```python
from build123d import *

# Parameters (mm, degrees)
EXTRUDE_1_DEPTH          = 10
EXTRUDE_2_DEPTH          = 10
EXTRUDE_3_DEPTH          = 900
SKETCH_4_W               = 40
SKETCH_4_H               = 15
EXTRUDE_4_DEPTH          = 45
CUT_EXTRUDE_1_DEPTH      = 975.114982946
CUT_EXTRUDE_1_DEPTH_BACK = 975.114982946
SKETCH_6_W               = 150
SKETCH_6_H               = 260
EXTRUDE_5_DEPTH          = 20
EXTRUDE_6_DEPTH          = 60
EXTRUDE_7_REACH          = 955.362
SKETCH_8_R               = 15
SKETCH_11_R              = 24
SKETCH_11_R_2            = 18
EXTRUDE_10_DEPTH         = 15
SKETCH_12_W              = 30
SKETCH_12_H              = 860
CUT_EXTRUDE_3_DEPTH      = 10
SKETCH_13_W              = 5
SKETCH_13_H              = 860
EXTRUDE_11_DEPTH         = 5
SKETCH_14_W              = 8
SKETCH_14_H              = 860
EXTRUDE_12_DEPTH         = 3
SKETCH_17_R              = 5
CUT_EXTRUDE_4_DEPTH      = 5
SKETCH_20_W              = 20
SKETCH_20_H              = 20
EXTRUDE_13_DEPTH         = 10
SKETCH_23_W              = 10
SKETCH_23_H              = 10
CUT_EXTRUDE_8_DEPTH      = 20


with BuildPart() as part:
    # 草图1 → 凸台-拉伸1 (new body)
    with BuildSketch(Plane(origin=(0, 0, 0), x_dir=(1, 0, 0), z_dir=(0, 1, 0))):
        Polygon((-150, 50), (-150, 150), (200, 150), (200, -150), (-150, -150), align=None)
    extrude(amount=EXTRUDE_1_DEPTH)

    # 草图2 → 凸台-拉伸2 (add)
    with BuildSketch(Plane(origin=(0, 10, 0), x_dir=(1, 0, 0), z_dir=(0, 1, 0))):
        with BuildLine():
            Line((-100, -20), (-100, 120))
            ThreePointArc((-100, 120), (-94.142135624, 134.142135624), (-80, 140))
            Line((-80, 140), (80, 140))
            ThreePointArc((80, 140), (94.142135624, 134.142135624), (100, 120))
            Line((100, 120), (100, -120))
            ThreePointArc((100, -120), (94.142135624, -134.142135624), (80, -140))
            Line((80, -140), (-80, -140))
            ThreePointArc((-80, -140), (-94.142135624, -134.142135624), (-100, -120))
            Line((-100, -120), (-100, -20))
        make_face()
    extrude(amount=EXTRUDE_2_DEPTH)

    # 草图3 → 凸台-拉伸3 (add)
    with BuildSketch(Plane(origin=(0, 20, 0), x_dir=(1, 0, 0), z_dir=(0, 1, 0))):
        Polygon((-50, 100), (-50, -100), (-50, -130), (-40, -130), (-40, 130), (-50, 130), align=None)
    extrude(amount=EXTRUDE_3_DEPTH)

    # 草图4 → 凸台-拉伸4 (add)
    with BuildSketch(Plane(origin=(0, 20, 0), x_dir=(1, 0, 0), z_dir=(0, 1, 0))):
        with Locations((-70, -92.5)):
            Rectangle(SKETCH_4_W, SKETCH_4_H)
        with Locations((-70, 92.5)):
            Rectangle(SKETCH_4_W, SKETCH_4_H)
    extrude(amount=EXTRUDE_4_DEPTH)

    # 草图5 → 切除-拉伸1 (cut, two sides: drawn at the far end of the back side and taken through both)
    with BuildSketch(Plane(origin=(0, 0, -100), x_dir=(-1, 0, 0), z_dir=(0, 0, -1)).offset(-CUT_EXTRUDE_1_DEPTH_BACK)):
        Polygon((90, 65), (90, 50), (50, 65), align=None)
    extrude(amount=CUT_EXTRUDE_1_DEPTH + CUT_EXTRUDE_1_DEPTH_BACK, mode=Mode.SUBTRACT)

    # 草图6 → 凸台-拉伸5 (add)
    with BuildSketch(Plane(origin=(0, 920, 0), x_dir=(1, 0, 0), z_dir=(0, 1, 0))):
        with Locations((25, 0)):
            Rectangle(SKETCH_6_W, SKETCH_6_H)
    extrude(amount=EXTRUDE_5_DEPTH)

    # 草图7 → 凸台-拉伸6 (add)
    with BuildSketch(Plane(origin=(-40, 0, 0), x_dir=(0, 0, -1), z_dir=(1, 0, 0))):
        Polygon((-95, 920), (-65, 920), (-65, 60), (-65, 20), (-95, 20), (-95, 60), align=None)
        Polygon((95, 920), (65, 920), (65, 60), (65, 20), (95, 20), (95, 60), align=None)
    extrude(amount=EXTRUDE_6_DEPTH)

    # 草图8 → 凸台-拉伸7 (add, up to next)
    with BuildSketch(Plane(origin=(0, 20, 0), x_dir=(1, 0, 0), z_dir=(0, 1, 0)), mode=Mode.PRIVATE) as extrude_7_sk1:
        with Locations(Location((0, 0, 0), (0, 0, 90))):
            Circle(SKETCH_8_R)
    extrude_7_tool1 = extrude(extrude_7_sk1.sketch, amount=EXTRUDE_7_REACH, mode=Mode.PRIVATE) - part.part
    add(extrude_7_tool1.solids().sort_by_distance((0, 20, 0))[0])

    # 草图11 → 凸台-拉伸10 (add)
    with BuildSketch(Plane.XZ.offset(-920)):
        with Locations(Location((0, 0, 0), (0, 0, 90))):
            Circle(SKETCH_11_R)
        with Locations(Location((0, 0, 0), (0, 0, 270))):
            Circle(SKETCH_11_R_2, mode=Mode.SUBTRACT)
    extrude(amount=EXTRUDE_10_DEPTH)

    # 草图12 → 切除-拉伸3 (cut)
    with BuildSketch(Plane(origin=(20, 0, 0), x_dir=(0, 0, -1), z_dir=(1, 0, 0))):
        with Locations((80, 490)):
            Rectangle(SKETCH_12_W, SKETCH_12_H)
        with Locations((-80, 490)):
            Rectangle(SKETCH_12_W, SKETCH_12_H)
    extrude(amount=-CUT_EXTRUDE_3_DEPTH, mode=Mode.SUBTRACT)

    # 草图13 → 凸台-拉伸11 (add)
    with BuildSketch(Plane(origin=(10, 0, 0), x_dir=(0, 0, -1), z_dir=(1, 0, 0))):
        with Locations((-92.5, 490)):
            Rectangle(SKETCH_13_W, SKETCH_13_H)
        with Locations((-67.5, 490)):
            Rectangle(SKETCH_13_W, SKETCH_13_H)
        with Locations((67.5, 490)):
            Rectangle(SKETCH_13_W, SKETCH_13_H)
        with Locations((92.5, 490)):
            Rectangle(SKETCH_13_W, SKETCH_13_H)
    extrude(amount=EXTRUDE_11_DEPTH)

    # 草图14 → 凸台-拉伸12 (add)
    with BuildSketch(Plane(origin=(15, 0, 0), x_dir=(0, 0, -1), z_dir=(1, 0, 0))):
        with Locations((-91, 490)):
            Rectangle(SKETCH_14_W, SKETCH_14_H)
        with Locations((-69, 490)):
            Rectangle(SKETCH_14_W, SKETCH_14_H)
        with Locations((69, 490)):
            Rectangle(SKETCH_14_W, SKETCH_14_H)
        with Locations((91, 490)):
            Rectangle(SKETCH_14_W, SKETCH_14_H)
    extrude(amount=EXTRUDE_12_DEPTH)

    # 草图17 → 切除-拉伸4 (cut)
    with BuildSketch(Plane(origin=(10, 0, 0), x_dir=(0, 0, -1), z_dir=(1, 0, 0))):
        with Locations((-80, 675)):
            Circle(SKETCH_17_R)
        with Locations((-80, 625)):
            Circle(SKETCH_17_R)
        with Locations((-80, 575)):
            Circle(SKETCH_17_R)
        with Locations((-80, 525)):
            Circle(SKETCH_17_R)
        with Locations((-80, 475)):
            Circle(SKETCH_17_R)
        with Locations((-80, 425)):
            Circle(SKETCH_17_R)
        with Locations((-80, 375)):
            Circle(SKETCH_17_R)
        with Locations((-80, 325)):
            Circle(SKETCH_17_R)
        with Locations((-80, 275)):
            Circle(SKETCH_17_R)
        with Locations((-80, 225)):
            Circle(SKETCH_17_R)
        with Locations((-80, 175)):
            Circle(SKETCH_17_R)
        with Locations((-80, 125)):
            Circle(SKETCH_17_R)
        with Locations((-80, 75)):
            Circle(SKETCH_17_R)
        with Locations((80, 675)):
            Circle(SKETCH_17_R)
        with Locations((80, 625)):
            Circle(SKETCH_17_R)
        with Locations((80, 575)):
            Circle(SKETCH_17_R)
        with Locations((80, 525)):
            Circle(SKETCH_17_R)
        with Locations((80, 475)):
            Circle(SKETCH_17_R)
        with Locations((80, 425)):
            Circle(SKETCH_17_R)
        with Locations((80, 375)):
            Circle(SKETCH_17_R)
        with Locations((80, 325)):
            Circle(SKETCH_17_R)
        with Locations((80, 275)):
            Circle(SKETCH_17_R)
        with Locations((80, 225)):
            Circle(SKETCH_17_R)
        with Locations((80, 175)):
            Circle(SKETCH_17_R)
        with Locations((80, 125)):
            Circle(SKETCH_17_R)
        with Locations((80, 75)):
            Circle(SKETCH_17_R)
        with Locations((-80, 725)):
            Circle(SKETCH_17_R)
        with Locations((-80, 775)):
            Circle(SKETCH_17_R)
        with Locations((-80, 825)):
            Circle(SKETCH_17_R)
        with Locations((-80, 875)):
            Circle(SKETCH_17_R)
        with Locations((80, 725)):
            Circle(SKETCH_17_R)
        with Locations((80, 775)):
            Circle(SKETCH_17_R)
        with Locations((80, 825)):
            Circle(SKETCH_17_R)
        with Locations((80, 875)):
            Circle(SKETCH_17_R)
    extrude(amount=-CUT_EXTRUDE_4_DEPTH, mode=Mode.SUBTRACT)

    # 草图20 → 凸台-拉伸13 (add)
    with BuildSketch(Plane(origin=(-40, 0, 0), x_dir=(0, 0, -1), z_dir=(1, 0, 0))):
        with Locations((-55, 215)):
            Rectangle(SKETCH_20_W, SKETCH_20_H)
        with Locations((55, 215)):
            Rectangle(SKETCH_20_W, SKETCH_20_H)
        with Locations((-55, 500)):
            Rectangle(SKETCH_20_W, SKETCH_20_H)
        with Locations((-55, 780)):
            Rectangle(SKETCH_20_W, SKETCH_20_H)
        with Locations((55, 500)):
            Rectangle(SKETCH_20_W, SKETCH_20_H)
        with Locations((55, 780)):
            Rectangle(SKETCH_20_W, SKETCH_20_H)
    extrude(amount=EXTRUDE_13_DEPTH)

    # 草图23 → 切除-拉伸8 (cut)
    with BuildSketch(Plane(origin=(-30, 0, 0), x_dir=(0, 0, -1), z_dir=(1, 0, 0))):
        with Locations((-55, 780)):
            Rectangle(SKETCH_23_W, SKETCH_23_H)
        with Locations((-55, 500)):
            Rectangle(SKETCH_23_W, SKETCH_23_H)
        with Locations((-55, 215)):
            Rectangle(SKETCH_23_W, SKETCH_23_H)
        with Locations((55, 215)):
            Rectangle(SKETCH_23_W, SKETCH_23_H)
        with Locations((55, 500)):
            Rectangle(SKETCH_23_W, SKETCH_23_H)
        with Locations((55, 780)):
            Rectangle(SKETCH_23_W, SKETCH_23_H)
    extrude(amount=-CUT_EXTRUDE_8_DEPTH, mode=Mode.SUBTRACT)


solid = part.part
```
Read the model definition and answer for the solid it produces. Units are mm, in the model's axes. A direction names the side the tool comes from. Give positions to 0.01 mm unless a question says otherwise; leave off trailing zeros. Write each loop counter-clockwise with the first axis right and the second up, starting at its lowest first coordinate (ties: lowest second). Pieces come first, ordered by that corner, then holes. Notation, with made-up numbers: (25.25, 9.5) - (73.25, 9.5) arc R7 cw to (73.25, 16.5) - close; hole circle Ø4 at (11, 62.5). An arc over 180 degrees is marked (long way). Write item = value, one per line. Start each with the question number.
Item 1: Find section C-C (x = -109.5). Give the vertices of the cut face in (y, z), then the cut area to 3 significant figures.
Item 2: Find section B-B (z = 0). Give the vertices of the cut face in (x, y), then the cut area to 3 significant figures.
Item 3: A tool of negligible diameter and unlimited length cuts with its end or side. For faces 1 (the flat face through (-42, 614, -130)), 2 (the flat face through (-30, 787, -55)), 3 (the flat face through (-10, 464, -95)), 4 (the flat face through (100, 930, 2)), 5 (the flat face through (-4, 920, -15)), from which of +Z, -Z, +X, -X, +Y, -Y can it reach the whole face along a straight path? Write none if from no direction.
Item 4: Find the intervals of material crossed by probe 1 along X at (y, z) = (913.75, 0); probe 2 along Y at (x, z) = (-10, -26); probe 3 along Z at (x, y) = (8.15, 375), in increasing order. Write a range as [from, to].
Item 5: The mould has two halves that part along Y. Classify faces 6 (the flat face through (-30, 208, -55)), 7 (the flat face through (24, 940, -2)), 8 (the flat face through (-42, 614, 130)): +Y half, -Y half, draft (parallel to the pull), parting line (faces both ways), or undercut.
Item 6: Each of these flat-tipped pins is pushed along its axis until it touches: P1, Ø13, axis at y = 625, z = 80, coming from the -X side; P2, Ø3, axis at y = 675, z = -82.5, coming from the +X side; P3, Ø10, axis at x = -99, z = -93.5, coming from the +Y side. Where does it stop, or does it pass through?
Response:
q1.outline = (0, -150) - (10, -150) - (10, 150) - (0, 150) - close
q1.area = 3,000 mm²
q2.outline = (-150, 0) - (200, 0) - (200, 10) - (100, 10) - (100, 20) - (15, 20) - (15, 920) - (18, 920) - (18, 905) - (24, 905) - (24, 920) - (100, 920) - (100, 940) - (-50, 940) - (-50, 20) - (-100, 20) - (-100, 10) - (-150, 10) - close; hole (-40, 20) - (-15, 20) - (-15, 920) - (-18, 920) - (-18, 905) - (-24, 905) - (-24, 920) - (-40, 920) - close
q2.area = 44,700 mm²
q3.face_1 = -Z, +X, -X, +Y
q3.face_2 = +X
q3.face_3 = -Z, +X
q3.face_4 = +Z, -Z, +X, +Y
q3.face_5 = none
q4.probe_1 = [-50, -40], [-24, -18], [-15, 15], [18, 24]
q4.probe_2 = [0, 20], [920, 940]
q4.probe_3 = [-95, -85], [-75, -65], [-12.59, 12.59], [65, 75], [85, 95]
q5.face_6 = undercut
q5.face_7 = +Y half
q5.face_8 = draft
q6.P1 = -50
q6.P2 = 5
q6.P3 = 20
